Autodesk Inventor part; units mm, degrees
ref_plane "YZ Plane" through (0, 0, 0) normal (1, 0, 0) x (0, 1, 0)
ref_plane "XZ Plane" through (0, 0, 0) normal (0, 1, 0) x (-1, 0, 0)
ref_plane "XY Plane" through (0, 0, 0) normal (0, 0, 1) x (1, 0, 0)
sketch "Esquisse1" plane through (0, 0, 0) normal (0, 1, 0) x (-1, 0, 0)
  circle A0 centre (0, 0) radius 14.075
  dimension "d0" = 28.15
extrude "Extrusion1" add sketch "Esquisse1" along normal blind 8
sketch "Esquisse2" plane through (0, 8, 0) normal (0, 1, 0) x (1, 0, 0)
  circle A0 centre (0, 0) radius 14.075
  circle A1 centre (0, 0) radius 17.5
  dimension "d3" = 35
extrude "Extrusion2" add sketch "Esquisse2" along normal blind 1 contours A0 | A1
sketch "Esquisse3" plane through (0, 0, 0) normal (0, -1, 0) x (1, 0, 0)
  circle A0 centre (0, 0) radius 14.075
  circle A1 centre (0, 0) radius 17.5
  dimension "d6" = 35
extrude "Extrusion3" add sketch "Esquisse3" along normal blind 1 contours A0 | A1
sketch "Esquisse4" plane through (0, -1, 0) normal (0, -1, 0) x (1, 0, 0)
  circle A0 centre (0, 0) radius 17.5
  circle A1 centre (0, 0) radius 11
  dimension "d9" = 22
extrude "Extrusion4" add sketch "Esquisse4" along normal blind 6 contours A1
sketch "Esquisse5" plane through (0, -7, 0) normal (0, -1, 0) x (1, 0, 0)
  circle A0 centre (0, 0) radius 11
  circle A1 centre (0, 0) radius 3
  dimension "d12" = 6
extrude "Extrusion5" cut sketch "Esquisse5" against normal through all contours A1
properties part number "poulie_rs_16T2p5s40-2"
Read the model definition and answer for the solid it produces. Units are mm, in the model's axes. A direction names the side the tool comes from. Coordinates: 2 decimals unless noted, no trailing zeros. Loops run counter-clockwise (first coordinate to the right, second up) from the corner with the lowest first, then second, coordinate; pieces in that order, holes last. Notation, with made-up numbers: (13, 59) -> (52, 59) arc R15 cw to (52, 68) -> close; hole circle Ø9 at (53.5, -7). An arc over 180 degrees is marked (long way). Return JSON: item names as keys, results as strings.
Item 1: Find section C-C (y = -3.5). Determine the outline of the cut face in (x, z), plus the area to 3 significant figures.
Answers:
{"outline": "circle Ø22 at (0, 0); hole circle Ø6 at (0, 0)", "area": "352 mm2"}
Item 2: Flat-ended cylindrical pins translate along their axes: P1, Ø8, axis at y = 3, z = 9.5, coming from the -X side; P2, Ø2, axis at x = -14, y = 1.5, coming from the -Z side. Find the tip coordinate at first contact, or state that the pin passes through.
Answers:
{"P1": "stops at x = -16.1", "P2": "stops at z = -5.39"}
Item 3: For a pull along Y with two mould halves and no side action, classify faces 1 (the cylindrical face through (3.05, 3.94, 13.74)), 2 (the flat face through (2.3, -7, -2.3)), 3 (the cylindrical face through (-3, 1, 0)) as +Y half, -Y half, draft (parallel to the pull), parting line (faces both ways), or undercut.
Answers:
{"face 1": "undercut", "face 2": "-Y half", "face 3": "draft"}
Item 4: For faces 4 (the cylindrical face through (-2.38, -3.96, 10.74)), 5 (the flat face through (-12, 8, -8)), 6 (the cylindrical face through (-13.887, 8.493, -10.648)), determine the directions among +Z, -Z, +X, -X, +Y, -Y from which every point of the face is accessible in a straight line to the end or side of a thin tool.
Answers:
{"face 4": "-Y", "face 5": "none", "face 6": "+Y, -Y"}
Item 5: Find section B-B (x = 0). Determine the outline of the cut face in (y, z) (3 decimals), plus the area to 3 significant figures.
Answers:
{"outline": "(-7, -11) -> (-1, -11) -> (-1, -17.5) -> (0, -17.5) -> (0, -14.075) -> (8, -14.075) -> (8, -17.5) -> (9, -17.5) -> (9, -3) -> (-7, -3) -> close; (-7, 3) -> (9, 3) -> (9, 17.5) -> (8, 17.5) -> (8, 14.075) -> (0, 14.075) -> (0, 17.5) -> (-1, 17.5) -> (-1, 11) -> (-7, 11) -> close", "area": "331 mm2"}
Item 6: Find the intervals of material crossed by probe 1 along Z at (x, y) = (0, -2.5); probe 2 along Y at (x, z) = (-11, 9); probe 3 along Z at (x, y) = (0, 5.75) (3 decimals), in increasing order.
Answers:
{"probe 1": "z = -11 to -3, 3 to 11", "probe 2": "y = -1 to 0, 8 to 9", "probe 3": "z = -14.075 to -3, 3 to 14.075"}
Item 7: Find section A-A (z = 0). Determine the outline of the cut face in (x, y) (3 decimals).
Answers:
{"outline": "(-17.5, -1) -> (-11, -1) -> (-11, -7) -> (-3, -7) -> (-3, 9) -> (-17.5, 9) -> (-17.5, 8) -> (-14.075, 8) -> (-14.075, 0) -> (-17.5, 0) -> close; (3, -7) -> (11, -7) -> (11, -1) -> (17.5, -1) -> (17.5, 0) -> (14.075, 0) -> (14.075, 8) -> (17.5, 8) -> (17.5, 9) -> (3, 9) -> close"}
Item 8: Find section D-D (z = -10). Determine the outline of the cut face in (x, y), plus the area to 3 significant figures.
Answers:
{"outline": "(-14.36, -1) -> (-4.58, -1) -> (-4.58, -7) -> (4.58, -7) -> (4.58, -1) -> (14.36, -1) -> (14.36, 0) -> (9.9, 0) -> (9.9, 8) -> (14.36, 8) -> (14.36, 9) -> (-14.36, 9) -> (-14.36, 8) -> (-9.9, 8) -> (-9.9, 0) -> (-14.36, 0) -> close", "area": "271 mm2"}
